Source: CAD feature listing. Evaluate the final solid. Frame: model axes, mm. A direction names the side the tool comes from. Give positions to 0.01 mm unless a question says otherwise; leave off trailing zeros. Loops run counter-clockwise (first coordinate to the right, second up) from the corner with the lowest first, then second, coordinate; pieces in that order, holes last. Notation, with made-up numbers: M 46,53 L 91,53 A27 ccw 91,80 Z; hole C -19.75,-10 d5. An arc over 180 degrees is marked long. Answer in a Markdown table with one row per item.
```python
from build123d import *

# Parameters (mm, degrees)
SKETCH1_W                = 1778
SKETCH1_H                = 127
BOSS_EXTRUDE1_DEPTH      = 127
SKETCH2_W                = 127
SKETCH2_H                = 127
BOSS_EXTRUDE2_DEPTH      = 508
SKETCH3_W                = 127
SKETCH3_H                = 127
BOSS_EXTRUDE3_DEPTH      = 508
BOSS_EXTRUDE4_DEPTH      = 431.8
BOSS_EXTRUDE4_DEPTH_BACK = 558.8
SKETCH4_R                = 6.35
BOSS_EXTRUDE5_DEPTH      = 508
BOSS_EXTRUDE5_DEPTH_BACK = 635
SKETCH6_R                = 6.35
BOSS_EXTRUDE7_DEPTH      = 12.7
BOSS_EXTRUDE8_DEPTH      = 12.7
SKETCH11_W               = 1016
SKETCH11_H               = 139.7
BOSS_EXTRUDE9_DEPTH      = 12.7
SKETCH12_W               = 1016
SKETCH12_H               = 139.7
BOSS_EXTRUDE10_DEPTH     = 12.7
SKETCH13_W               = 127
SKETCH13_H               = 127
BOSS_EXTRUDE11_DEPTH     = 127
SKETCH15_W               = 63.5
SKETCH15_H               = 63.5
CUT_EXTRUDE1_DEPTH       = 63.5


with BuildPart() as part:
    # Sketch1 → Boss-Extrude1 (new body)
    with BuildSketch(Plane.XY):
        Rectangle(SKETCH1_W, SKETCH1_H)
    extrude(amount=BOSS_EXTRUDE1_DEPTH)

    # Sketch2 → Boss-Extrude2 (add)
    with BuildSketch(Plane.XY.offset(127)):
        Rectangle(SKETCH2_W, SKETCH2_H)
    extrude(amount=BOSS_EXTRUDE2_DEPTH)

    # Sketch3 → Boss-Extrude3 (add)
    with BuildSketch(Plane(origin=(0, 0, 0), x_dir=(-1, 0, 0), z_dir=(0, 0, -1))):
        Rectangle(SKETCH3_W, SKETCH3_H)
    extrude(amount=BOSS_EXTRUDE3_DEPTH)

    # Sketch4 → Boss-Extrude4 (add, two sides: drawn at the far end of the back side and taken through both)
    with BuildSketch(Plane.XY.offset(127).offset(-BOSS_EXTRUDE4_DEPTH_BACK)):
        with Locations((-762, 0)):
            Circle(SKETCH4_R)
    extrude(amount=BOSS_EXTRUDE4_DEPTH + BOSS_EXTRUDE4_DEPTH_BACK)

    # Sketch6 → Boss-Extrude5 (add, two sides: drawn at the far end of the back side and taken through both)
    with BuildSketch(Plane.XY.offset(127).offset(-BOSS_EXTRUDE5_DEPTH_BACK)):
        with Locations((762, 0)):
            Circle(SKETCH6_R)
    extrude(amount=BOSS_EXTRUDE5_DEPTH + BOSS_EXTRUDE5_DEPTH_BACK)

    # Sketch9 → Boss-Extrude7 (add)
    with BuildSketch(Plane(origin=(0, 63.5, 0), x_dir=(1, 0, 0), z_dir=(0, 1, 0))):
        with BuildLine():
            Line((-63.5, 508), (-63.5, -635))
            Line((-63.5, -635), (381, -635))
            ThreePointArc((381, -635), (740.210244843, -486.210244843), (889, -127))
            Line((889, -127), (889, 0))
            ThreePointArc((889, 0), (740.210244843, 359.210244843), (381, 508))
            Line((381, 508), (-63.5, 508))
        make_face()
    extrude(amount=BOSS_EXTRUDE7_DEPTH)

    # Sketch10 → Boss-Extrude8 (add)
    with BuildSketch(Plane(origin=(0, 63.5, 0), x_dir=(1, 0, 0), z_dir=(0, 1, 0))):
        with BuildLine():
            Line((-63.5, -635), (-889, -127))
            Line((-889, -127), (-889, 0))
            Line((-889, 0), (-63.5, 508))
            Line((-63.5, 508), (381, 508))
            ThreePointArc((381, 508), (740.210244843, 359.210244843), (889, 0))
            Line((889, 0), (889, -127))
            ThreePointArc((889, -127), (740.210244843, -486.210244843), (381, -635))
            Line((381, -635), (-63.5, -635))
        make_face()
    extrude(amount=BOSS_EXTRUDE8_DEPTH)

    # Sketch11 → Boss-Extrude9 (add)
    with BuildSketch(Plane(origin=(0, 0, -508), x_dir=(-1, 0, 0), z_dir=(0, 0, -1))):
        with Locations((0, 6.35)):
            Rectangle(SKETCH11_W, SKETCH11_H)
    extrude(amount=BOSS_EXTRUDE9_DEPTH)

    # Sketch12 → Boss-Extrude10 (add)
    with BuildSketch(Plane.XY.offset(635)):
        with Locations((0, 6.35)):
            Rectangle(SKETCH12_W, SKETCH12_H)
    extrude(amount=BOSS_EXTRUDE10_DEPTH)

    # Sketch13 → Boss-Extrude11 (add)
    with BuildSketch(Plane(origin=(0, 76.2, 0), x_dir=(1, 0, 0), z_dir=(0, 1, 0))):
        Polygon((-889, 330.2), (-889, 0), (-1016, 0), (-1016, 203.2), align=None)
        Polygon((-1016, -330.2), (-889, -457.2), (-889, -127), (-1016, -127), align=None)
        with Locations((-952.5, -63.5)):
            Rectangle(SKETCH13_W, SKETCH13_H)
    extrude(amount=-BOSS_EXTRUDE11_DEPTH)

    # Sketch15 → Cut-Extrude1 (cut)
    with BuildSketch(Plane(origin=(0, 76.2, 0), x_dir=(1, 0, 0), z_dir=(0, 1, 0))):
        with Locations((762, -63.5)):
            Rectangle(SKETCH15_W, SKETCH15_H)
    extrude(amount=-CUT_EXTRUDE1_DEPTH, mode=Mode.SUBTRACT)


solid = part.part
```
1) Material intervals for L1, parallel to Z at x = 491, y = -23; L2, parallel to X at y = 62.5, z = -164.5; L3, parallel to Y at x = 768.5, z = 145, sorted ascending.
Reply:
| item | result |
|---|---|
| L1 | z = -520.7 to -508, 0 to 127, 635 to 647.7 |
| L2 | x = -1016 to -889, -63.5 to 63.5 |
| L3 | y = 63.5 to 76.2 |
2) Section D-D, the plane x = -551. Return loops of the section in (y, z).
Reply:
| item | result |
|---|---|
| outline | M -63.5,0 L 63.5,0 L 63.5,-208 L 76.2,-208 L 76.2,335 L 63.5,335 L 63.5,127 L -63.5,127 Z |
3) Pull-direction query (X, two-part tool) for faces 1 (the flat face through (-482.028, 69.761, -250.444)), 2 (the flat face through (-289, 7, 635)), 3 (the flat face through (-953.4, 13.6, -265.8)); classes: released by +X, released by -X, zero draft, split by the parting line, or undercut.
Reply:
| item | result |
|---|---|
| face 1 | undercut |
| face 2 | zero draft |
| face 3 | released by -X |
4) Set-up query: faces 4 (the flat face through (-63.5, -1, 377)), 5 (the flat face through (762, 45, 31.75)), 6 (the flat face through (-889, 14, -163)). Return all of +Z, -Z, +X, -X, +Y, -Y with unobstructed straight access to the full face (end or side cutting, diameter ignored); none if empty.
Reply:
| item | result |
|---|---|
| face 4 | -Y |
| face 5 | +Y |
| face 6 | -Z, +Y, -Y |
5) Pin query (flat end, axial travel): pin 1 Ø4 at (y, z) = (-33, 373.5) entering from +X; pin 2 Ø5 at (x, y) = (549.5, 5.5) entering from +Z; pin 3 Ø10 at (y, z) = (27.5, -513) entering from -X. Return the tip coordinate at first contact, or that it passes through.
Reply:
| item | result |
|---|---|
| pin 1 | stops at x = 63.5 |
| pin 2 | stops at z = 127 |
| pin 3 | stops at x = -508 |
6) Section B-B, the plane x = 456.5. Return loops of the section in (y, z), then the cut area to 3 significant figures.
Reply:
| item | result |
|---|---|
| outline | M -63.5,-520.7 L 76.2,-520.7 L 76.2,-508 L -63.5,-508 Z; M -63.5,0 L 63.5,0 L 63.5,-502.36 L 76.2,-502.36 L 76.2,629.36 L 63.5,629.36 L 63.5,127 L -63.5,127 Z; M -63.5,635 L 76.2,635 L 76.2,647.7 L -63.5,647.7 Z |
| area | 34,100 mm² |
7) Section C-C, the plane z = -264. Return loops of the section in (x, y).
Reply:
| item | result |
|---|---|
| outline | M -955.2,-50.8 L -889,-50.8 L -889,76.2 L -955.2,76.2 Z; C -762,0 d12.7; M -460,63.5 L -63.5,63.5 L -63.5,-63.5 L 63.5,-63.5 L 63.5,63.5 L 815.01,63.5 L 815.01,76.2 L -460,76.2 Z; C 762,0 d12.7 |
8) Section A-A, the plane y = 45. Return loops of the section in (x, z), then the cut area to 3 significant figures.
Reply:
| item | result |
|---|---|
| outline | M -1016,-203.2 L -889,-330.2 L -889,0 L -63.5,0 L -63.5,-508 L -508,-508 L -508,-520.7 L 508,-520.7 L 508,-508 L 63.5,-508 L 63.5,0 L 889,0 L 889,127 L 63.5,127 L 63.5,635 L 508,635 L 508,647.7 L -508,647.7 L -508,635 L -63.5,635 L -63.5,127 L -889,127 L -889,457.2 L -1016,330.2 Z; hole M 730.25,31.75 L 793.75,31.75 L 793.75,95.25 L 730.25,95.25 Z |
| area | 460,000 mm² |
